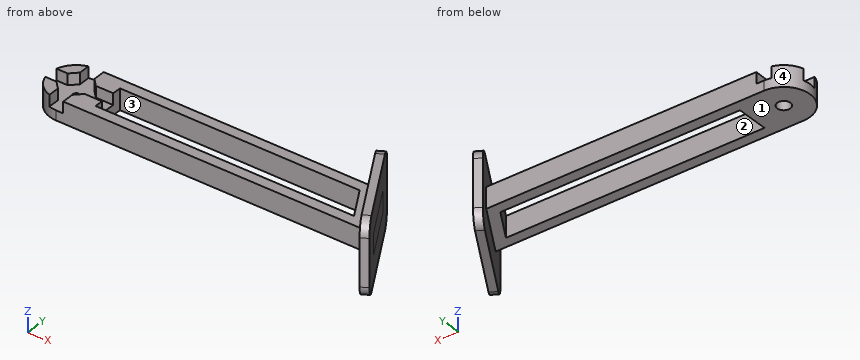
```python
from build123d import *

# Parameters (mm, degrees)
BOSS_EXTRU_1_DEPTH       = 8
ESQUISSE13_R             = 4
ENL_V_MAT_EXTRU_9_DEPTH  = 4.3
ENL_V_MAT_EXTRU_10_DEPTH = 4.3
ESQUISSE15_R             = 2.5
ENL_V_MAT_EXTRU_11_DEPTH = 3.4
ENL_V_MAT_EXTRU_12_REACH = 6.6
ESQUISSE16_R             = 1.25
ESQUISSE17_W             = 10
ESQUISSE17_H             = 20
ENL_V_MAT_EXTRU_13_DEPTH = 10
ENL_V_MAT_EXTRU_15_DEPTH = 10
ESQUISSE20_W             = 28
ESQUISSE20_H             = 43.094010768
BOSS_EXTRU_2_DEPTH       = 3
ENL_V_MAT_EXTRU_16_REACH = 20
CONG_1_R                 = 5


with BuildPart() as part:
    # Esquisse1 → Boss.-Extru.1 (new body)
    with BuildSketch(Plane.XY):
        with BuildLine():
            Line((0, 0), (120, 0))
            ThreePointArc((120, 0), (130, 10), (120, 20))
            Line((120, 20), (0, 20))
            ThreePointArc((0, 20), (-10, 10), (0, 0))
        make_face()
    extrude(amount=BOSS_EXTRU_1_DEPTH)

    # Esquisse13 → Enlèv. mat.-Extru.9 (cut)
    with BuildSketch(Plane.XY.offset(8)):
        with Locations((0, 10)):
            Circle(ESQUISSE13_R)
    extrude(amount=-ENL_V_MAT_EXTRU_9_DEPTH, mode=Mode.SUBTRACT)

    # Esquisse14 → Enlèv. mat.-Extru.10 (cut)
    with BuildSketch(Plane.XY.offset(8)):
        Polygon((2.655377087, 4.544050257), (2.655377087, -2.008601379), (-2.844622913, -1.912365766), (-2.844622913, 4.640285869), (-5.455949743, 7.344622913), (-12.008601379, 7.344622913), (-11.912365766, 12.844622913), (-5.359714131, 12.844622913), (-2.655377087, 15.455949743), (-2.655377087, 22.008601379), (2.844622913, 21.912365766), (2.844622913, 15.359714131), (5.455949743, 12.655377087), (12.008601379, 12.655377087), (11.912365766, 7.155377087), (5.359714131, 7.155377087), align=None)
    extrude(amount=-ENL_V_MAT_EXTRU_10_DEPTH, mode=Mode.SUBTRACT)

    # Esquisse15 → Enlèv. mat.-Extru.11 (cut)
    with BuildSketch(Plane(origin=(0, 0, 0), x_dir=(-1, 0, 0), z_dir=(0, 0, -1))):
        with Locations((0, 10)):
            Circle(ESQUISSE15_R)
    extrude(amount=-ENL_V_MAT_EXTRU_11_DEPTH, mode=Mode.SUBTRACT)

    # Esquisse16 → Enlèv. mat.-Extru.12 (cut, up to next)
    with BuildSketch(Plane(origin=(0, 0, 3.4), x_dir=(-1, 0, 0), z_dir=(0, 0, -1)), mode=Mode.PRIVATE) as enl_v_mat_extru_12_sk1:
        with Locations((0, 10)):
            Circle(ESQUISSE16_R)
    enl_v_mat_extru_12_tool1 = extrude(enl_v_mat_extru_12_sk1.sketch, amount=-ENL_V_MAT_EXTRU_12_REACH, mode=Mode.PRIVATE) & part.part
    add(enl_v_mat_extru_12_tool1.solids().sort_by_distance((0, 10, 3.4))[0], mode=Mode.SUBTRACT)

    # Esquisse17 → Enlèv. mat.-Extru.13 (cut)
    with BuildSketch(Plane.XY.offset(8)):
        with Locations((125, 10)):
            Rectangle(ESQUISSE17_W, ESQUISSE17_H)
    extrude(amount=-ENL_V_MAT_EXTRU_13_DEPTH, mode=Mode.SUBTRACT)

    # Esquisse19 → Enlèv. mat.-Extru.15 (cut)
    with BuildSketch(Plane(origin=(0, 0, 0), x_dir=(-1, 0, 0), z_dir=(0, 0, -1))):
        Polygon((-131.547005384, 0), (-120, 0), (-108.452994616, 20), (-120, 20), align=None)
    extrude(amount=-ENL_V_MAT_EXTRU_15_DEPTH, mode=Mode.SUBTRACT)

    # Esquisse20 → Boss.-Extru.2 (add)
    with BuildSketch(Plane(origin=(90, 51.961524227, 0), x_dir=(0, 0, -1), z_dir=(0.866025404, 0.5, 0))):
        with Locations((-4, -48.452994616)):
            Rectangle(ESQUISSE20_W, ESQUISSE20_H)
    extrude(amount=-BOSS_EXTRU_2_DEPTH)

    # Esquisse21 → Enlèv. mat.-Extru.16 (cut, up to next)
    with BuildSketch(Plane.XY.offset(8), mode=Mode.PRIVATE) as enl_v_mat_extru_16_sk1:
        Polygon((11.857154921, 4), (109.607695155, 4), (102.679491924, 16), (12.06712353, 16), align=None)
    enl_v_mat_extru_16_tool1 = extrude(enl_v_mat_extru_16_sk1.sketch, amount=-ENL_V_MAT_EXTRU_16_REACH, mode=Mode.PRIVATE) & part.part
    add(enl_v_mat_extru_16_tool1.solids().sort_by_distance((59.074082, 9.924208, 8))[0], mode=Mode.SUBTRACT)

    # Congé1
    cong_1_edges = [part.edges().sort_by_distance(p)[0] for p in [
        (123.700961894, -9.410254038, 18),
        (102.153956511, 27.910254038, 18),
        (102.153956511, 27.910254038, -10),
        (123.700961894, -9.410254038, -10),
    ]]
    fillet(cong_1_edges, radius=CONG_1_R)


solid = part.part
```
Input: part model. Units: mm. Frame: model coordinates. Face numbers are marked on the shaded views. Coordinates: 2 decimals unless noted, no trailing zeros. Order: outer loops, then holes, each group sorted by start corner. A loop starts at its lowest first (then second) coordinate and runs counter-clockwise, first axis right, second up. Notation, with made-up numbers: (-11, -14) - (24, -14) arc R16 ccw to (24, 5) - close; hole circle Ø7 at (-31, 16.5). An arc over 180 degrees is marked (long way). Return JSON: item names as keys, results as strings.
Q1. Cut plane D-D (x = 112). Return loops of the section in (y, z), then the cut area to 3 significant figures.
The answers:
{"outline": "(0, 0) - (7.86, 0) - (7.86, -10) - (13.86, -10) - (13.86, 18) - (7.86, 18) - (7.86, 8) - (0, 8) - close", "area": "231 mm2"}
Q2. Cut plane A-A (z = 6.5). Return loops of the section in (x, y).
The answers:
{"outline": "(-9.64, 7.34) arc R10 ccw to (-2.84, 0.41) - (-2.84, 4.64) - (-5.46, 7.34) - close; (-9.59, 12.84) - (-5.36, 12.84) - (-2.66, 15.46) - (-2.66, 19.64) arc R10 ccw to start; (2.66, 0) - (116.54, 0) - (122.4, -10.16) - (125, -8.66) - (103.45, 28.66) - (100.85, 27.16) - (104.99, 20) - (2.84, 20) - (2.84, 15.36) - (5.46, 12.66) - (12.01, 12.66) - (12.07, 16) - (102.68, 16) - (109.61, 4) - (11.86, 4) - (11.91, 7.16) - (5.36, 7.16) - (2.66, 4.54) - close"}
Q3. Ray query, probe 1 along Y at (x, z) = (0, 3.65); probe 2 along X at (y, z) = (15.5, 4.5); probe 3 along Z at (x, y) = (8, 13). Return the intervals inside material, ascending.
The answers:
{"probe 1": "y = 0 to 8.75, 11.25 to 20", "probe 2": "x = -8.35 to -2.66, 2.84 to 12.06, 102.97 to 111.05", "probe 3": "z = 0 to 8"}
Q4. Draft query along Y for the marked faces 1, 2, 3 and 4. Return one class per face: +Y half, -Y half, draft (parallel to the pull), parting line (faces both ways), or undercut.
The answers:
{"face 1": "draft", "face 2": "undercut", "face 3": "undercut", "face 4": "parting line"}
Q5. Cut plane C-C (y = 10). Return loops of the section in (x, z).
The answers:
{"outline": "(-10, 0) - (-2.5, 0) - (-2.5, 3.4) - (-1.25, 3.4) - (-1.25, 3.7) - (-10, 3.7) - close; (1.25, 3.4) - (2.5, 3.4) - (2.5, 0) - (11.96, 0) - (11.96, 3.7) - (1.25, 3.7) - close; (106.14, 0) - (110.76, 0) - (110.76, -10) - (114.23, -10) - (114.23, 18) - (110.76, 18) - (110.76, 8) - (106.14, 8) - close"}
Q6. First-contact query: pin 1 (2 mm diameter, centred on y = 19, z = -2, fed in from -X); pin 2 (8 mm diameter, centred on y = 13, z = 9, fed in from -X); pin 3 (2 mm diameter, centred on x = 82.5, z = -1.5, fed in from +Y); pin 4 (9 mm diameter, centred on x = 44.5, z = 5, fed in from -Y). Flat tips, straight axial feed; report the tip coordinate or a pass-through.
The answers:
{"pin 1": "stops at x = 104.99", "pin 2": "stops at x = -9.59", "pin 3": "passes through", "pin 4": "stops at y = 0"}
Q7. Cut plane B-B (x = 74.5). Return loops of the section in (y, z).
The answers:
{"outline": "(0, 0) - (4, 0) - (4, 8) - (0, 8) - close; (16, 0) - (20, 0) - (20, 8) - (16, 8) - close"}
